```python
from build123d import *

# Parameters (mm, degrees)
F1_DEPTH = 25.4
F2_R     = 9.525
F3_DEPTH = 91.186
F4_R     = 9.2433485979
F5_DEPTH = 31.75
F6_SIZE  = 6.35
F7_SIZE  = 6.35


with BuildPart() as f1:
    # F0 (on Top) → F1 (new body)
    with BuildSketch(Plane.XY):
        Polygon((25.4, 15.875), (-12.7, 15.875), (-12.7, 25.4), (-38.1, 25.4), (-38.1, -25.4), (-12.7, -25.4), (-12.7, -15.875), (25.4, -15.875), align=None)
    extrude(amount=F1_DEPTH)

    # F2 (on face) → F3 (cut)
    with BuildSketch(Plane.XZ.offset(25.4)):
        with Locations((-25.4, 12.7)):
            Circle(F2_R)
    extrude(amount=-F3_DEPTH, mode=Mode.SUBTRACT)

    # F4 (on face) → F5 (cut)
    with BuildSketch(Plane.YZ.offset(25.4)):
        with Locations((0, 12.7)):
            Circle(F4_R)
    extrude(amount=-F5_DEPTH, mode=Mode.SUBTRACT)

    # F6
    f6_edges = [f1.edges().sort_by_distance(p)[0] for p in [
        (-12.7, 15.875, 12.7),
        (-12.7, -15.875, 12.7),
    ]]
    chamfer(f6_edges, length=F6_SIZE)

    # F7
    f7_edges = [f1.edges().sort_by_distance(p)[0] for p in [
        (-12.7, -23.8125, 25.4),
        (-9.525, -19.05, 25.4),
        (9.525, -15.875, 25.4),
        (9.525, 15.875, 25.4),
        (-9.525, 19.05, 25.4),
        (-12.7, 23.8125, 25.4),
        (-38.1, 0, 25.4),
        (9.525, 15.875, 0),
        (-9.525, 19.05, 0),
        (-12.7, 23.8125, 0),
        (-38.1, 0, 0),
        (-12.7, -23.8125, 0),
        (-9.525, -19.05, 0),
        (9.525, -15.875, 0),
    ]]
    chamfer(f7_edges, length=F7_SIZE)


solid = f1.part
```
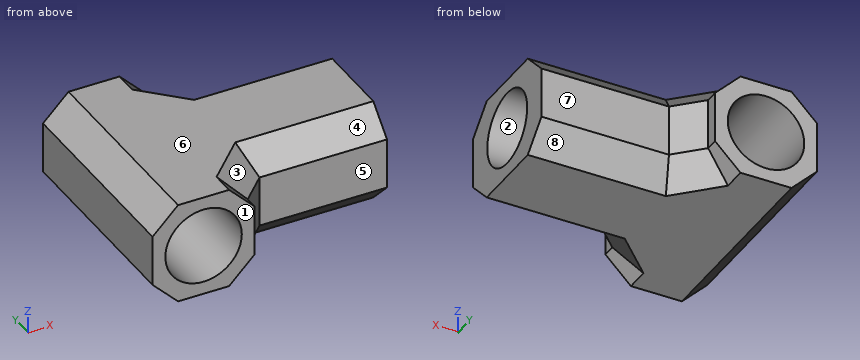
Verification items for the finished model (mm, model axes). Face numbers are marked on the shaded views. A direction names the side the tool comes from. Give positions to 0.01 mm unless a question says otherwise; leave off trailing zeros. Order: outer loops, then holes, each group sorted by start corner. A loop starts at its lowest first (then second) coordinate and runs counter-clockwise, first axis right, second up. Notation, with made-up numbers: (46, 24) -> (95, 24) arc R31 cw to (95, 57) -> close; hole circle Ø8 at (-21.5, 33). An arc over 180 degrees is marked (long way). One line per item, written item: value.
(1) Sectioned sample at D-D on x = 14. Record the cut outline in (y, z) (3 decimals), then the cut area to 3 significant figures.
Final values:
outline: (-15.875, 6.35) -> (-9.525, 0) -> (9.525, 0) -> (15.875, 6.35) -> (15.875, 19.05) -> (9.525, 25.4) -> (-9.525, 25.4) -> (-15.875, 19.05) -> close; hole circle Ø18.487 at (0, 12.7)
area: 457 mm^2
(2) Sectioned sample at C-C on z = 12.7. Record the cut outline in (x, y) (3 decimals).
Final values:
outline: (-38.1, -25.4) -> (-34.925, -25.4) -> (-34.925, 25.4) -> (-38.1, 25.4) -> close; (-15.875, -25.4) -> (-12.7, -25.4) -> (-12.7, -22.225) -> (-6.35, -15.875) -> (25.4, -15.875) -> (25.4, -9.243) -> (-6.35, -9.243) -> (-6.35, 9.243) -> (25.4, 9.243) -> (25.4, 15.875) -> (-6.35, 15.875) -> (-12.7, 22.225) -> (-12.7, 25.4) -> (-15.875, 25.4) -> close
(3) Tool access check on the marked faces 4, 5, 6, 7 and 8. Record the directions out of +Z, -Z, +X, -X, +Y, -Y that give a thin tool (end or side, any length) a straight path to the whole face; none if there is none.
Final values:
face 4: +Z, +X, -Y
face 5: +Z, -Z, +X, -Y
face 6: +Z, +X, -X, +Y, -Y
face 7: +Z, -Z, +X, +Y
face 8: -Z, +X, +Y
(4) Draft check along Z on the marked faces 1, 2 and 3. Enter one of: pulls with the +Z half, pulls with the -Z half, needs draft (parallel to the pull), parting line crosses it, or undercut.
Final values:
face 1: needs draft
face 2: undercut
face 3: pulls with the +Z half
(5) Gauge pin test, flat ends, axial feed: pin 1 (1 mm diameter, centred on y = -23, z = 14, fed in from +X); pin 2 (10 mm diameter, centred on x = -7.5, y = -19, fed in from -Z); pin 3 (15 mm diameter, centred on y = 0, z = 12.7, fed in from +X); pin 4 (6 mm diameter, centred on x = -5.5, y = 11.5, fed in from +Z). Record the tip position at first contact, or that the pin passes through.
Final values:
pin 1: x = -12.7
pin 2: z = 2.75
pin 3: x = -6.35
pin 4: z = 25.4
(6) Sectioned sample at A-A on x = -25.4. Record the cut outline in (y, z) (3 decimals), then the cut area to 3 significant figures.
Final values:
outline: (-25.4, 0) -> (25.4, 0) -> (25.4, 3.175) -> (-25.4, 3.175) -> close; (-25.4, 22.225) -> (25.4, 22.225) -> (25.4, 25.4) -> (-25.4, 25.4) -> close
area: 323 mm^2
(7) Sectioned sample at B-B on y = 0. Record the cut outline in (x, z) (3 decimals).
Final values:
outline: (-38.1, 6.35) -> (-31.75, 0) -> (25.4, 0) -> (25.4, 3.457) -> (-6.35, 3.457) -> (-6.35, 21.943) -> (25.4, 21.943) -> (25.4, 25.4) -> (-31.75, 25.4) -> (-38.1, 19.05) -> close; hole circle Ø19.05 at (-25.4, 12.7)
(8) Scan lines: line 1 along Z through (x, y) = (-25.5, -5.5); line 2 along Z through (x, y) = (3.5, 0); line 3 along X through (y, z) = (15, 14.25). Record each from-to range of solid material in increasing order. Write a range as [from, to].
Final values:
line 1: [0, 3.18], [22.22, 25.4]
line 2: [0, 3.46], [21.94, 25.4]
line 3: [-38.1, -34.8], [-16, 25.4]
